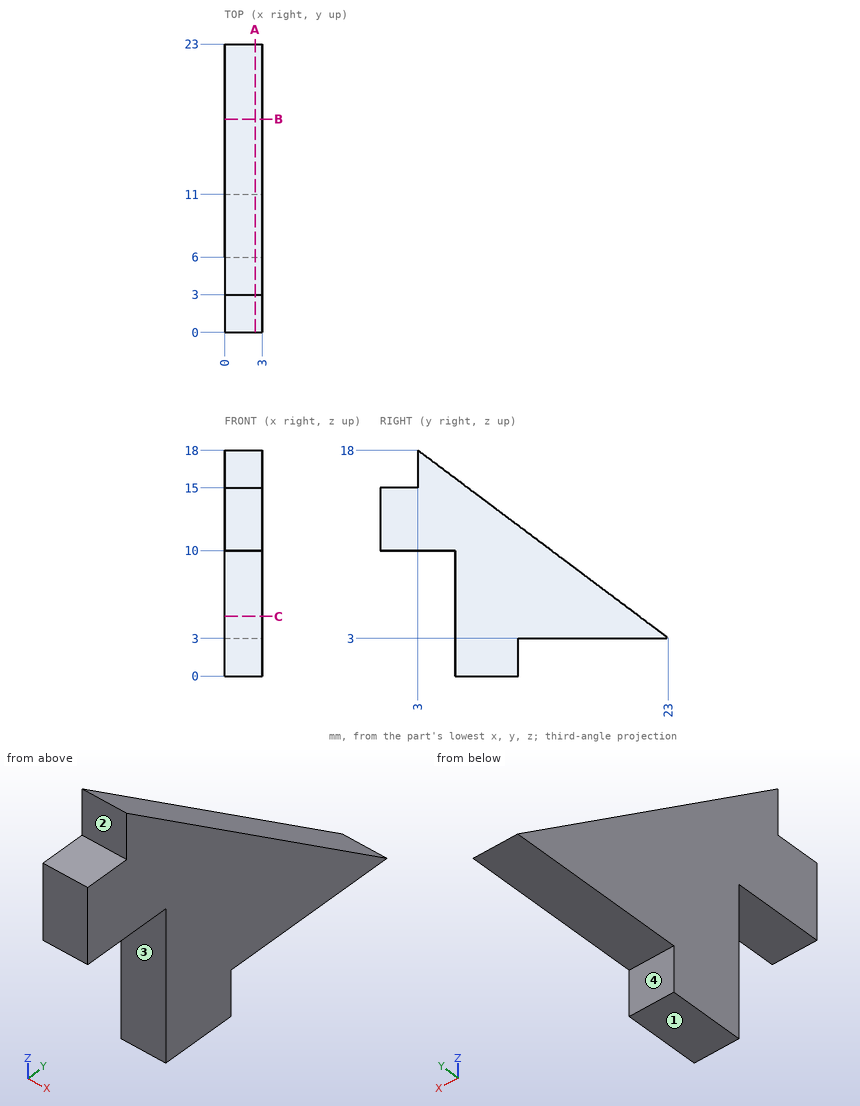
The drawing under review shows one solid part. Ordinate dimensions are in mm from its lowest x, y, z. A direction names the side the tool comes from. Round coordinates to 2 decimals unless told otherwise and drop trailing zeros. Write each loop counter-clockwise with the first axis right and the second up, starting at its lowest first coordinate (ties: lowest second). Pieces come first, ordered by that corner, then holes.
(1) We need section C-C on z = 4.75. Give the boundary of the cut face in (x, y), and give its area (3 significant figures).
(2) We need section B-B on y = 17. Give the boundary of the cut face in (x, z).
(3) Machinability: for the marked faces 1, 2, 3 and 4, which of the approach directions +Z, -Z, +X, -X, +Y, -Y give a long, thin tool a straight path to every point of the face, cutting with its end or side? Answer none if there is none.
(4) Insertion check: pin 1 (1 mm diameter, centred on x = 1, z = 7.5, fed in from -Y); pin 2 (0.9 mm diameter, centred on x = 1.5, y = 3.5, fed in from -Z); pin 3 (0.9 mm diameter, centred on x = 1.5, z = 1, fed in from +Y). Each pin has a flat end and moves straight along its axis. Give the tip position at first contact, or say it passes through.
(5) Wall thickness on L1, parallel to Y at x = 1.2, z = 1.25; L2, parallel to Y at x = 1.55, z = 6.75; L3, parallel to Z at x = 0.85, y = 2.5: over which ranges is each line inside the solid? List them lowest first.
(6) We need section A-A on x = 2.45. Give the boundary of the cut face in (y, z), and give its area (3 significant figures).
Findings below:
1. outline: (0, 6) - (3, 6) - (3, 20.67) - (0, 20.67) - close
1. area: 44.0 mm2
2. outline: (0, 3) - (3, 3) - (3, 7.5) - (0, 7.5) - close
3. face 1: -Z, +X, -X, +Y, -Y
3. face 2: +Z, +X, -X, -Y
3. face 3: -Z, +X, -X, -Y
3. face 4: -Z, +X, -X, +Y
4. pin 1: stops at y = 6
4. pin 2: stops at z = 10
4. pin 3: stops at y = 11
5. L1: y = 6 to 11
5. L2: y = 6 to 18
5. L3: z = 10 to 15
6. outline: (0, 10) - (6, 10) - (6, 0) - (11, 0) - (11, 3) - (23, 3) - (3, 18) - (3, 15) - (0, 15) - close
6. area: 159 mm2
